Geometry check sheet. Reference: the model listing, model coordinates, mm. Round coordinates to 2 decimals unless told otherwise and drop trailing zeros. Write each loop counter-clockwise with the first axis right and the second up, starting at its lowest first coordinate (ties: lowest second). Pieces come first, ordered by that corner, then holes. Notation, with made-up numbers: M -7,22.25 L 1,22.25 A24 cw 1,48.25 Z; hole C 76.5,63 d7. An arc over 180 degrees is marked long. Put each result on its own line as item: value. Start each with the question number.
(1) Section check C-C on x = -19. Record the cut outline in (y, z).
(2) Section check A-A on z = 0. Record the cut outline in (x, y), then the cut area to 4 significant figures.
(3) Mould release check, pull along Y, two halves, no side actions. Record for faces 1 (the cylindrical face through (0, 2, 0)), 2 (the flat face through (27.5, 2, 2)), 3 (the cylindrical face through (-0.378, -3.905, -0.867)): pulls with the +Y half, pulls with the -Y half, needs draft (parallel to the pull), parting line crosses it, or undercut.
(4) Gauge pin test, flat ends, axial feed: pin 1 (3 mm diameter, centred on x = -10, z = -2.5, fed in from +Y); pin 2 (4 mm diameter, centred on x = 7, y = -2.5, fed in from +Z); pin 3 (3 mm diameter, centred on x = 14, y = 3, fed in from -Z). Record the tip position at first contact, or that the pin passes through.
(5) Material ranges on probe 1 along Y at (x, z) = (-6, 0); probe 2 along Y at (x, z) = (23, 0.75), recorded low to high.
Solid Edge part; units mm, degrees
sketch "Sketch1" plane through (0, 0, 0) normal (0, -1, 0) x (1, 0, 0)
  line L0 (27.5, 0) -> (27.5, 4)
  line L1 (27.5, 4) -> (-27.5, 4)
  line L2 (-27.5, 4) -> (-27.5, 0)
  dimension "D1" = 27.5
revolve "RevolvedProtrusion1" add sketch "Sketch1" angle 360 about axis through (-32.5, 0, 0) along (1, 0, 0)
chamfer "Chamfer1" distance 0.5 angle 45 2 edges at (27.5, 0, -4) (-27.5, 0, -4)
hole "Hole_1" at (-27.5, 0, 0) direction (1, 0, 0) diameter 4 depth 60 tip angle 118
properties material "Polyethylene, low density"
Answers follow:
1. outline: C 0,0 d8; hole C 0,0 d4
2. outline: M -27.5,-3.5 L -27,-4 L 27,-4 L 27.5,-3.5 L 27.5,-2 L -27.5,-2 Z; M -27.5,2 L 27.5,2 L 27.5,3.5 L 27,4 L -27,4 L -27.5,3.5 Z
2. area: 219.5 mm^2
3. face 1: undercut
3. face 2: needs draft
3. face 3: parting line crosses it
4. pin 1: stops at y = 3.87
4. pin 2: stops at z = 3.97
4. pin 3: stops at z = -3.71
5. probe 1: y = -4 to -2, 2 to 4
5. probe 2: y = -3.93 to -1.85, 1.85 to 3.93
